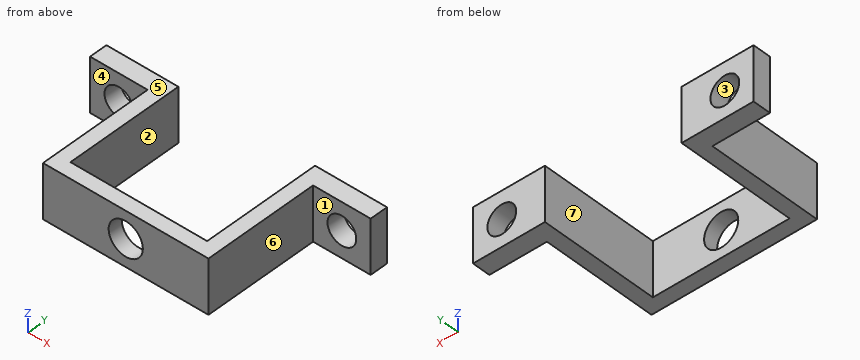
from build123d import *

# Parameters (mm, degrees)
RESSALTO_EXTRUS_O1_DEPTH   = 7.5
CORTE_EXTRUS_O2_DEPTH      = 55.27936993
CORTE_EXTRUS_O2_DEPTH_BACK = 55.27936993
ESBO_O3_R                  = 4.75
CORTE_EXTRUS_O3_DEPTH      = 52.002450921
CORTE_EXTRUS_O3_DEPTH_BACK = 52.002450921
ESBO_O4_R                  = 4


with BuildPart() as part:
    # Esboço1 → Ressalto-extrusão1 (new, symmetric)
    with BuildSketch(Plane.XY):
        Polygon((19, 0), (-19, 0), (-19, 33), (-39, 33), (-39, 28), (-23, 28), (-23, -4), (23, -4), (23, 28), (39, 28), (39, 33), (19, 33), align=None)
    extrude(amount=RESSALTO_EXTRUS_O1_DEPTH, both=True)

    # Esboço3 → Corte-extrusão2 (cut, two sides: drawn at the far end of the back side and taken through both)
    with BuildSketch(Plane(origin=(0, -4, 0), x_dir=(-1, 0, 0), z_dir=(0, -1, 0)).offset(-CORTE_EXTRUS_O2_DEPTH_BACK)):
        with Locations(Location((0, 0, 0), (0, 0, 90))):
            Circle(ESBO_O3_R)
    extrude(amount=CORTE_EXTRUS_O2_DEPTH + CORTE_EXTRUS_O2_DEPTH_BACK, mode=Mode.SUBTRACT)

    # Esboço4 → Corte-extrusão3 (cut, two sides: drawn at the far end of the back side and taken through both)
    with BuildSketch(Plane(origin=(0, 28, 0), x_dir=(-1, 0, 0), z_dir=(0, -1, 0)).offset(-CORTE_EXTRUS_O3_DEPTH_BACK)):
        with Locations(Location((31, 0.149250584, 0), (0, 0, 90))):
            Circle(ESBO_O4_R)
        with Locations(Location((-31, 0.149250584, 0), (0, 0, 90))):
            Circle(ESBO_O4_R)
    extrude(amount=CORTE_EXTRUS_O3_DEPTH + CORTE_EXTRUS_O3_DEPTH_BACK, mode=Mode.SUBTRACT)


solid = part.part
Design review of the part built by this model. Coordinates are the model's own, in mm. Face numbers are marked on the shaded views. A direction names the side the tool comes from. Round coordinates to 2 decimals unless told otherwise and drop trailing zeros. Write each loop counter-clockwise with the first axis right and the second up, starting at its lowest first coordinate (ties: lowest second). Pieces come first, ordered by that corner, then holes. Notation, with made-up numbers: M 48,43 L 89,43 A26 ccw 89,69 Z; hole C 80.25,82.25 d9. An arc over 180 degrees is marked long. One line per item, written item: value. Start each with the question number.
1. Take a section at B-B on y = 25. State the section outline as (x, z) points, then the cut area to 3 significant figures.
2. Clearance check with flat-ended pins moving along their axes: P1, Ø9, axis at x = 31, z = -0.15, coming from the +Y side; P2, Ø7.5, axis at x = -8, z = 1, coming from the +Y side; P3, Ø7.5, axis at x = 30, z = 3.5, coming from the -Y side; P4, Ø2, axis at y = 17.5, z = 5, coming from the -X side. State where each tip first meets the part, or that it passes through.
3. Take a section at A-A on x = 0. State the section outline as (y, z) points.
4. Draft analysis for pull direction X (two halves, no side actions). For the marked faces 5, 6 and 7, state which applies: pulls with the +X half, pulls with the -X half, needs draft (parallel to the pull), parting line crosses it, or undercut.
5. Take a section at D-D on z = -5.75. State the section outline as (x, y) points.
6. For the marked faces 1, 2, 3 and 4, list the 3-axis set-ups (+Z, -Z, +X, -X, +Y, -Y) from which the entire face can be reached by the end or side of a thin tool; tool diameter is ignored.
7. To check wall thickness, follow probe 1 along X at (y, z) = (31.5, -0.25); probe 2 along X at (y, z) = (7.5, 0); probe 3 along X at (y, z) = (31.5, 5). State the ranges of each line that lie inside material, in increasing order. Write a range as from..to.
8. Take a section at C-C on z = -2. State the section outline as (x, y) points, then the cut area to 3 significant figures.
Computed:
1. outline: M -23,-7.5 L -19,-7.5 L -19,7.5 L -23,7.5 Z; M 19,-7.5 L 23,-7.5 L 23,7.5 L 19,7.5 Z
1. area: 120 mm²
2. P1: stops at y = 33
2. P2: stops at y = 0
2. P3: stops at y = 28
2. P4: stops at x = -23
3. outline: M -4,-7.5 L 0,-7.5 L 0,-4.75 L -4,-4.75 Z; M -4,4.75 L 0,4.75 L 0,7.5 L -4,7.5 Z
4. face 5: needs draft
4. face 6: pulls with the +X half
4. face 7: undercut
5. outline: M -39,28 L -23,28 L -23,-4 L 23,-4 L 23,28 L 39,28 L 39,33 L 19,33 L 19,0 L -19,0 L -19,33 L -39,33 Z
6. face 1: +Z, -Z, +X, -Y
6. face 2: +Z, -Z, +Y
6. face 3: +Y, -Y
6. face 4: +Z, -Z, -X, -Y
7. probe 1: x = -39..-35, -27..-19, 19..27, 35..39
7. probe 2: x = -23..-19, 19..23
7. probe 3: x = -39..-19, 19..39
8. outline: M -39,28 L -34.55,28 L -34.55,33 L -39,33 Z; M -27.45,28 L -23,28 L -23,-4 L -4.31,-4 L -4.31,0 L -19,0 L -19,33 L -27.45,33 Z; M 4.31,-4 L 23,-4 L 23,28 L 27.45,28 L 27.45,33 L 19,33 L 19,0 L 4.31,0 Z; M 34.55,28 L 39,28 L 39,33 L 34.55,33 Z
8. area: 503 mm²
